Here's how the part is built. I have some questions about the finished solid (model axes, mm). A direction names the side the tool comes from. Round coordinates to 2 decimals unless told otherwise and drop trailing zeros. Write each loop counter-clockwise with the first axis right and the second up, starting at its lowest first coordinate (ties: lowest second). Pieces come first, ordered by that corner, then holes. Notation, with made-up numbers: (76.25, -30) - (86.25, -30) arc R24 ccw to (86.25, -2) - close; hole circle Ø7 at (-3.75, 23). An arc over 180 degrees is marked (long way). One line per question, with ' | ' between items. Start each with the question number.
(1) Will these pins go through, and if not, where does the flat tip stop? pin 1 (6 mm diameter, centred on y = 52.76, z = 57.24, fed in from +X); pin 2 (1 mm diameter, centred on y = 2.5, z = 35.5, fed in from -X); pin 3 (7.5 mm diameter, centred on x = 42.5, y = -54, fed in from -Z); pin 4 (5 mm diameter, centred on x = 12.5, y = -57.5, fed in from +Z).
(2) Thinking about a two-plate mould opening in Y: for faces 4 (the flat face through (0, 75, 21)), 5 (the flat face through (57, -1, 43)), 6 (the flat face through (62, 60, 75)), which applies, pulls with the +Y half, pulls with the -Y half, needs draft (parallel to the pull), parting line crosses it, or undercut?
(3) If I drill on L1, parallel to Y at x = -44.5, z = 29; L2, parallel to Z at x = -12, y = 1; L3, parallel to X at y = -53, z = 35, over which ranges is the centre line in solid material (lowest first)?
(4) For faces 1 (the cylindrical face through (-3.681, -1.115, 9.506)), 2 (the flat face through (-49.52, -49.29, 2.46)), 3 (the flat face through (62, -60, 75)), which set-ups out of +Z, -Z, +X, -X, +Y, -Y let a thin tool reach every point of the face, with its end or its side?
(5) Imagine slicing it at C-C (z = 49.5). Write out the boundary of the cut face in (x, y), plus the area to 3 significant figures.
(6) Imagine slicing it at B-B (x = -28). Write out the boundary of the cut face in (y, z).
(7) Imagine slicing it at A-A (z = 68.5). Write out the boundary of the cut face in (x, y).
Autodesk Fusion 360 part; units mm, degrees
sketch "Sketch1" plane through (0, 0, 0) normal (0, 0, 1) x (1, 0, 0)
  line L0 (65, -75) -> (-65, -75)
  line L1 (-65, -75) -> (-65, 75)
  line L2 (-65, 75) -> (65, 75)
  line L3 (65, 75) -> (65, -75)
  line L4 (65, -75) -> (-65, 75) construction
  line L5 (-65, -75) -> (65, 75) construction
  dimension "d1" = 130
  dimension "d2" = 150
extrude "Extrude1" add sketch "Sketch1" along normal blind 75
sketch "Sketch2" plane through (65, 0, 0) normal (1, 0, 0) x (0, 1, 0)
  line L0 (-75, 0) -> (75, 0)
  line L1 (75, 0) -> (75, 75)
  line L2 (75, 75) -> (-75, 75)
  line L3 (-75, 75) -> (-75, 0)
  line L4 (0, 0) -> (0, 10)
  line L5 (0, 10) -> (0, 110)
  circle A0 centre (0, 110) radius 100.5
  circle A1 centre (0, 110) radius 74.615
  line L6 (0, 110) -> (52.7608, 57.2392)
  line L7 (0, 110) -> (74.615, 110) construction
  line L8 (0, 110) -> (-52.7608, 57.2392)
  line L9 (0, 110) -> (74.615, 110) construction
  circle A2 centre (52.7608, 57.2392) radius 5.2
  circle A3 centre (-52.7608, 57.2392) radius 5.2
  circle A4 centre (0, 110) radius 57.5
  dimension "d5" = 10
  dimension "d6" = 100
  dimension "d7" = 201
  dimension "d8" = 149.23
  dimension "d9" = 45
  dimension "d10" = 135
  dimension "d11" = 10.4
  dimension "d12" = 10.4
  dimension "d13" = 115
extrude "Extrude2" cut sketch "Sketch2" against normal blind 130 contours L2 L6 L8 A4 | L2 L8 A4 | L2 L5 L8 A4 | L2 L5 L6 A4 | L2 L5 L8 | L2 L6 A4 | L2 L5 L6
extrude "Extrude3" cut sketch "Sketch2" against normal blind 122 from surface at -8 contours L2 L3 L4 L5 A0 A1 A3 | L1 L2 L4 L5 A0 A1 A2 | L2 A1 L8 A3 A4 | L5 A1 L8 A3 A4 | L5 A1 L6 A2 A4 | A1 L8 A3 | A1 A3 | L2 A1 L6 A2 A4 | A1 L8 A3 | A1 L6 A2 | A1 A2 | A1 L6 A2
extrude "Extrude4" cut sketch "Sketch2" against normal blind 10 contours A1 L8 A3 | A1 A3 | A1 L8 A3 | A1 L6 A2 | A1 A2 | A1 L6 A2
fillet "Fillet1" radius 2 16 edges at (-65, 75, 21.5513) (-65, -75, 21.5513) (0, -75, 0) (0, 75, 0) (-4, -75, 43.1027) (-4, 75, 43.1027) (57, 60.3104, 75) (57, 75, 59.0513) (57, -75, 59.0513) (57, -60.3104, 75) (-65, 0, 9.5) (-65, 0, 0) (61, -75, 75) (61, 75, 75) (61, 45.6207, 75) (61, -45.6207, 75)
fillet "Fillet2" radius 3 5 edges at (57.5858, -74.4142, 39.4611) (57, -72.228, 39.8919) (57, 0, 9.5) (57, 72.228, 39.8919) (57.5858, 74.4142, 39.4611)
sketch "Sketch3" plane through (0, 0, 0) normal (0, 0, -1) x (1, 0, 0)
  line L0 (-63, -73) -> (65, -73)
  line L1 (65, -73) -> (65, 73)
  line L2 (65, 73) -> (-63, 73)
  line L3 (-63, 73) -> (-63, -73)
  line L4 (-63, 73) -> (-43, 73)
  line L5 (-43, 73) -> (-43, 53)
  line L6 (-38.6582, 45.5068) -> (-34.3398, 53.0135)
  line L7 (-34.3398, 53.0135) -> (-38.6816, 60.5067)
  line L8 (-38.6816, 60.5067) -> (-47.3418, 60.4932)
  line L9 (-47.3418, 60.4932) -> (-51.6602, 52.9865)
  line L10 (-51.6602, 52.9865) -> (-47.3184, 45.4933)
  line L11 (-47.3184, 45.4933) -> (-38.6582, 45.5068)
  line L12 (65, 73) -> (45, 73)
  line L13 (45, 73) -> (45, 53)
  line L14 (49.3301, 45.5) -> (53.6603, 53)
  line L15 (53.6603, 53) -> (49.3301, 60.5)
  line L16 (49.3301, 60.5) -> (40.6699, 60.5)
  line L17 (40.6699, 60.5) -> (36.3397, 53)
  line L18 (36.3397, 53) -> (40.6699, 45.5)
  line L19 (40.6699, 45.5) -> (49.3301, 45.5)
  line L20 (-63, -73) -> (-63, -53)
  line L21 (-63, -53) -> (-43, -53)
  line L22 (-38.6699, -60.5) -> (-34.3397, -53)
  line L23 (-34.3397, -53) -> (-38.6699, -45.5)
  line L24 (-38.6699, -45.5) -> (-47.3301, -45.5)
  line L25 (-47.3301, -45.5) -> (-51.6603, -53)
  line L26 (-51.6603, -53) -> (-47.3301, -60.5)
  line L27 (-47.3301, -60.5) -> (-38.6699, -60.5)
  line L28 (65, -73) -> (45, -73)
  line L29 (45, -73) -> (45, -53)
  line L30 (49.3301, -60.5) -> (53.6603, -53)
  line L31 (53.6603, -53) -> (49.3301, -45.5)
  line L32 (49.3301, -45.5) -> (40.6699, -45.5)
  line L33 (40.6699, -45.5) -> (36.3397, -53)
  line L34 (36.3397, -53) -> (40.6699, -60.5)
  line L35 (40.6699, -60.5) -> (49.3301, -60.5)
  point P0 (-43, 53)
  point P1 (45, 53)
  point P2 (-43, -53)
  point P3 (45, -53)
  dimension "d45" = 20
  dimension "d46" = 20
  dimension "d47" = 7.5
  dimension "d48" = 20
  dimension "d49" = 20
  dimension "d50" = 7.5
  dimension "d51" = 20
  dimension "d52" = 20
  dimension "d53" = 7.5
  dimension "d54" = 20
  dimension "d55" = 20
  dimension "d56" = 7.5
extrude "Extrude5" cut sketch "Sketch3" against normal blind 5 contours L30 L31 L32 L33 L34 L35 | L14 L15 L16 L17 L18 L19 | L6 L7 L8 L9 L10 L11 | L22 L23 L24 L25 L26 L27
Check sheet entries:
1) pin 1: through | pin 2: x = 57 | pin 3: z = 5 | pin 4: z = 29.38
2) face 4: pulls with the +Y half | face 5: undercut | face 6: needs draft
3) L1: -75 to -59.49, 59.49 to 75 | L2: 0 to 9.5 | L3: 57 to 65
4) face 1: +Z, -X | face 2: -Z | face 3: +Z, +X, -X, +Y, -Y
5) outline: (57, -73) arc R2 ccw to (59, -75) - (65, -75) - (65, 75) - (59, 75) arc R2 ccw to (57, 73) - close | area: 1,200 mm^2
6) outline: (-75, 2) arc R2 ccw to (-73, 0) - (73, 0) arc R2 ccw to (75, 2) - (75, 38.05) arc R2 ccw to (71.58, 39.45) arc R100.5 cw to (-71.58, 39.45) arc R2 ccw to (-75, 38.05) - close
7) outline: (57, -73) arc R2 ccw to (59, -75) - (65, -75) - (65, -39.8) - (57, -39.8) - close; (57, 39.8) - (65, 39.8) - (65, 75) - (59, 75) arc R2 ccw to (57, 73) - close
